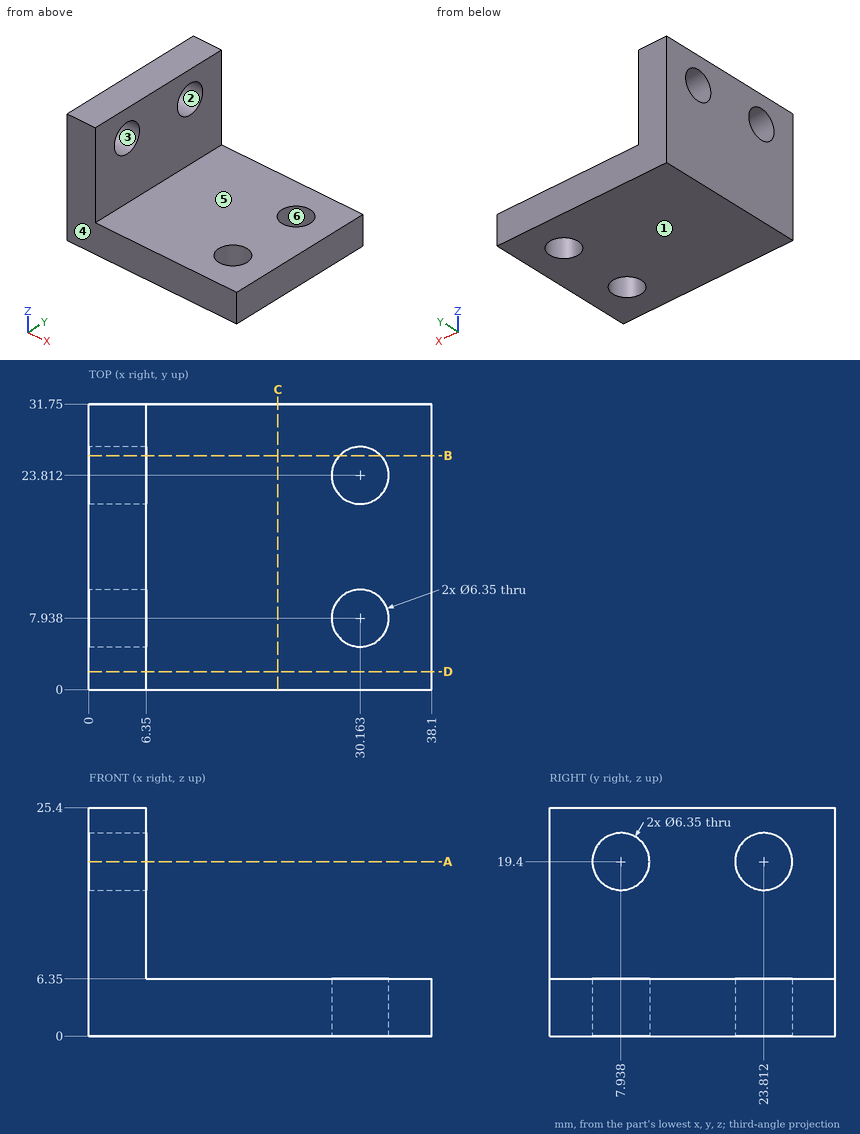
Source: three-view drawing plus pictorial views. Frame: mm from the lowest corner of the part. A direction names the side the tool comes from. Round coordinates to 2 decimals unless told otherwise and drop trailing zeros. Order: outer loops, then holes, each group sorted by start corner. A loop starts at its lowest first (then second) coordinate and runs counter-clockwise, first axis right, second up. Notation, with made-up numbers: (-34.5, -11) - (6.5, -11) arc R11 ccw to (6.5, 8) - close; hole circle Ø4 at (-0.75, 26). An arc over 180 degrees is marked (long way). Answer in a Markdown table with one row per item.
Item 1: Section query D-D (y = 2). Return the cut outline in (x, z).
Model answer:
| item | result |
|---|---|
| outline | (0, 0) - (38.1, 0) - (38.1, 6.35) - (6.35, 6.35) - (6.35, 25.4) - (0, 25.4) - close |
Item 2: Line query: line 1 (X direction, y = 8, z = 3.5); line 2 (Z direction, x = 30.5, y = 13); line 3 (X direction, y = 9.5, z = 3.75) (1 decimal). Output: solid intervals per line, ascending.
Model answer:
| item | result |
|---|---|
| line 1 | x = 0 to 26.99, 33.34 to 38.1 |
| line 2 | z = 0 to 6.35 |
| line 3 | x = 0 to 27.4, 32.9 to 38.1 |
Item 3: Section query A-A (z = 19.4). Return the cut outline in (x, y), then the cut area to 3 significant figures.
Model answer:
| item | result |
|---|---|
| outline | (0, 0) - (6.35, 0) - (6.35, 4.76) - (0, 4.76) - close; (0, 11.11) - (6.35, 11.11) - (6.35, 20.64) - (0, 20.64) - close; (0, 26.99) - (6.35, 26.99) - (6.35, 31.75) - (0, 31.75) - close |
| area | 121 mm² |
Item 4: Mould query, pull axis Z, two halves, no side actions, for the marked faces 1, 2, 3 and 4. Classes: released by +Z, released by -Z, zero draft, split by the parting line, or undercut.
Model answer:
| item | result |
|---|---|
| face 1 | released by -Z |
| face 2 | undercut |
| face 3 | undercut |
| face 4 | zero draft |
Item 5: Section query B-B (y = 26). Return the cut outline in (x, z).
Model answer:
| item | result |
|---|---|
| outline | (0, 0) - (27.86, 0) - (27.86, 6.35) - (6.35, 6.35) - (6.35, 17.1) - (0, 17.1) - close; (0, 21.7) - (6.35, 21.7) - (6.35, 25.4) - (0, 25.4) - close; (32.46, 0) - (38.1, 0) - (38.1, 6.35) - (32.46, 6.35) - close |
Item 6: Reachability of the marked faces 5 and 6 from +Z, -Z, +X, -X, +Y, -Y: full face, straight path, thin tool, end or side. Return the list, or none.
Model answer:
| item | result |
|---|---|
| face 5 | +Z, +X, +Y, -Y |
| face 6 | +Z, -Z |
Item 7: Pin query (flat end, axial travel): pin 1 (8.5 mm diameter, centred on x = 30.16, y = 23.81, fed in from +Z); pin 2 (4 mm diameter, centred on y = 27, z = 22.5, fed in from +X); pin 3 (5 mm diameter, centred on y = 7.94, z = 19.4, fed in from +X). Return the tip coordinate at first contact, or that it passes through.
Model answer:
| item | result |
|---|---|
| pin 1 | stops at z = 6.35 |
| pin 2 | stops at x = 6.35 |
| pin 3 | passes through |
Item 8: Section query C-C (x = 21). Return the cut outline in (y, z), then the cut area to 3 significant figures.
Model answer:
| item | result |
|---|---|
| outline | (0, 0) - (31.75, 0) - (31.75, 6.35) - (0, 6.35) - close |
| area | 202 mm² |
